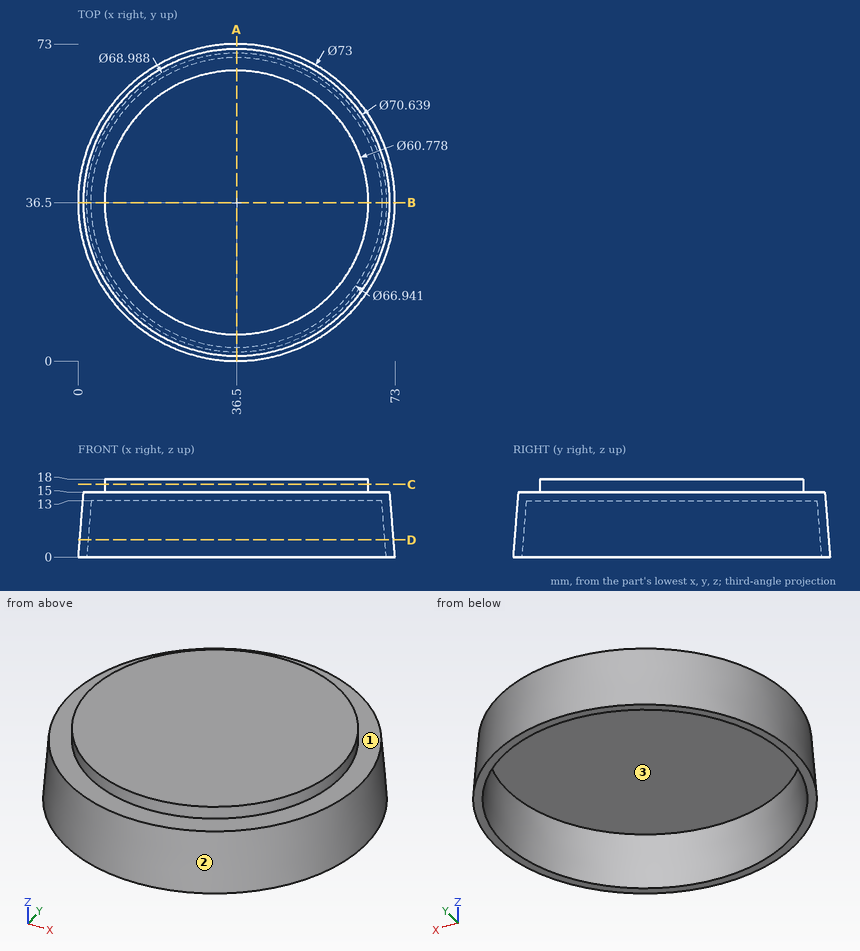
Print and shaded views of the part. All mm, measured from the part's lowest x, y and z. Round coordinates to 2 decimals unless told otherwise and drop trailing zeros. Order: outer loops, then holes, each group sorted by start corner. A loop starts at its lowest first (then second) coordinate and runs counter-clockwise, first axis right, second up.
Q1. Slice it at A-A (x = 36.5). Write the cut outline in (y, z).
Q2. Slice it at D-D (z = 4). Write the cut outline in (x, y) (1 decimal).
Q3. Slice it at C-C (z = 16.75). Write the cut outline in (x, y).
Q4. Wall check: L1, parallel to Z at x = 67.5, y = 42; L2, parallel to Z at x = 56, y = 54; L3, parallel to Y at x = 31, z = 10 (1 decimal). Give the ranges that are in metal, low to high.
Q5. Drop flat-ended pins along their axis: pin 1 (3 mm diameter, centred on x = 49.5, y = 44, fed in from -Z); pin 2 (4 mm diameter, centred on y = 30.5, z = 12.5, fed in from +X); pin 3 (1 mm diameter, centred on x = 55, z = 12, fed in from -Y). Give the stop position or say it passes through.
Q6. Two-plate mould, pull along Y, no slides. Class the marked faces 1, 2 and 3: pulls with the +Y half, pulls with the -Y half, needs draft (parallel to the pull), parting line crosses it, or undercut.
Results below:
1. outline: (0, 0) - (2.01, 0) - (3.03, 13) - (69.97, 13) - (70.99, 0) - (73, 0) - (71.82, 15) - (66.89, 15) - (66.89, 18) - (6.11, 18) - (6.11, 15) - (1.18, 15) - close
2. outline: circle Ø72.4 at (36.5, 36.5); hole circle Ø68.4 at (36.5, 36.5)
3. outline: circle Ø60.78 at (36.5, 36.5)
4. L1: z = 13 to 15
4. L2: z = 13 to 18
4. L3: y = 1.2 to 3.2, 69.8 to 71.8
5. pin 1: stops at z = 13
5. pin 2: stops at x = 71.84
5. pin 3: stops at y = 5.83
6. face 1: needs draft
6. face 2: parting line crosses it
6. face 3: undercut
